Check sheet for the modelled part. Datum: model origin and axes. Units: mm. A direction names the side the tool comes from. Coordinates: 2 decimals unless noted, no trailing zeros. Write each loop counter-clockwise with the first axis right and the second up, starting at its lowest first coordinate (ties: lowest second). Pieces come first, ordered by that corner, then holes. Notation, with made-up numbers: M -8.5,-31.75 L 0.5,-31.75 A28 cw 0.5,-12.75 Z; hole C -18.5,6.25 d5. An arc over 180 degrees is marked long. Answer as CSV lines item,"result".
from build123d import *

# Parameters (mm, degrees)
BOSS_EXTRUDE1_DEPTH = 20
SKETCH2_R           = 5
CUT_EXTRUDE1_DEPTH  = 20
SKETCH3_W           = 70
SKETCH3_H           = 20
SKETCH3_R           = 5
BOSS_EXTRUDE2_DEPTH = 14.55
SKETCH4_W           = 30
SKETCH4_H           = 10
BOSS_EXTRUDE3_DEPTH = 30
SKETCH5_R           = 5
CUT_EXTRUDE2_DEPTH  = 20


with BuildPart() as part:
    # Sketch1 → Boss-Extrude1 (new body)
    with BuildSketch(Plane.XY):
        Polygon((-125, -8.78), (125, -8.78), (125, 8.78), (-125, 8.78), (-125, 5), (-100, 5), (-100, -5), (-125, -5), align=None)
    extrude(amount=BOSS_EXTRUDE1_DEPTH)

    # Sketch2 → Cut-Extrude1 (cut, symmetric)
    with BuildSketch(Plane.XZ.offset(-5)):
        with Locations((-115, 10)):
            Circle(SKETCH2_R)
        with Locations((0, 10)):
            Circle(SKETCH2_R)
        with BuildLine():
            Line((-115, 20), (-115, 22.029141536))
            Line((-115, 22.029141536), (-130, 22.029141536))
            Line((-130, 22.029141536), (-130, -2.19309391))
            Line((-130, -2.19309391), (-115, -2.19309391))
            Line((-115, -2.19309391), (-115, 0))
            ThreePointArc((-115, 0), (-125, 10), (-115, 20))
        make_face()
    extrude(amount=CUT_EXTRUDE1_DEPTH, both=True, mode=Mode.SUBTRACT)

    # Sketch3 → Boss-Extrude2 (add)
    with BuildSketch(Plane.XZ.offset(8.78)):
        with Locations((0, 10)):
            Rectangle(SKETCH3_W, SKETCH3_H)
        with Locations((0, 10)):
            Circle(SKETCH3_R, mode=Mode.SUBTRACT)
    extrude(amount=BOSS_EXTRUDE2_DEPTH)

    # Sketch4 → Boss-Extrude3 (add)
    with BuildSketch(Plane.XZ.offset(8.78)):
        with Locations((110, 10)):
            Rectangle(SKETCH4_W, SKETCH4_H)
    extrude(amount=BOSS_EXTRUDE3_DEPTH)

    # Sketch5 → Cut-Extrude2 (cut)
    with BuildSketch(Plane.XY.offset(15)):
        with Locations((110, -23.78)):
            Circle(SKETCH5_R)
    extrude(amount=-CUT_EXTRUDE2_DEPTH, mode=Mode.SUBTRACT)


solid = part.part
1) Tool access check on faces 4 (the face through (106, -20, 5)), 5 (the face through (-81, -8.78, 10)), 6 (the face through (-109.5, -5, 9.9)), 7 (the face through (-125, 7, 10)). Record the directions out of +Z, -Z, +X, -X, +Y, -Y that give a thin tool (end or side, any length) a straight path to the whole face; none if there is none.
Answer key:
face 4,"-Z, +X, -Y"
face 5,"+Z, -Z, -X, -Y"
face 6,"+Z, -Z, -X"
face 7,"-X, +Y, -Y"
2) Section check D-D, the plane y = 1. Record the boundary of the cut face in (x, z), plus the area to 3 significant figures.
Answer key:
outline,"M -100,0 L 125,0 L 125,20 L -100,20 Z; hole C 0,10 d10"
area,"4,420 mm2"
3) Mould release check, pull along Y, two halves, no side actions. Record for faces 1 (the face through (-100, 0, 10)), 2 (the face through (0, -23.33, 17)), 3 (the face through (106, -20, 15)): pulls with the +Y half, pulls with the -Y half, needs draft (parallel to the pull), parting line crosses it, or undercut.
Answer key:
face 1,"undercut"
face 2,"pulls with the -Y half"
face 3,"needs draft"
4) Section check B-B, the plane x = 0. Record the boundary of the cut face in (y, z), plus the area to 3 significant figures.
Answer key:
outline,"M -23.33,0 L 8.78,0 L 8.78,5 L -23.33,5 Z; M -23.33,15 L 8.78,15 L 8.78,20 L -23.33,20 Z"
area,"321 mm2"
5) Section check C-C, the plane z = 2.5. Record the boundary of the cut face in (x, y).
Answer key:
outline,"M -121.61,-8.78 L -35,-8.78 L -35,-23.33 L 35,-23.33 L 35,-8.78 L 125,-8.78 L 125,8.78 L -121.61,8.78 L -121.61,5 L -100,5 L -100,-5 L -121.61,-5 Z"
6) Thickness scan on line 1 along X through (y, z) = (6.5, 10.5); line 2 along Y through (x, z) = (-103, 7.25); line 3 along Y through (x, z) = (110, 11.25). Record the ranges inside material, lowest first.
Answer key:
line 1,"x = -124.99 to -119.97, -110.03 to -4.97, 4.97 to 125"
line 2,"y = -8.78 to -5, 5 to 8.78"
line 3,"y = -38.78 to -28.78, -18.78 to 8.78"
7) Section check A-A, the plane y = -11. Record the boundary of the cut face in (x, z).
Answer key:
outline,"M -35,0 L 35,0 L 35,20 L -35,20 Z; M 95,5 L 125,5 L 125,15 L 95,15 Z; hole C 0,10 d10"
8) Depth check by flat-ended pin: P1, Ø9, axis at x = 104.5, y = -19, coming from the -Z side; P2, Ø8, axis at y = -9.5, z = 5, coming from the -X side; P3, Ø2, axis at x = 56.5, y = -11.5, coming from the +Z side; P4, Ø24, axis at x = 107, y = -31, coming from the +Z side. Enter the tip coordinate at first touch or a pass-through.
Answer key:
P1,"stops at z = 5"
P2,"stops at x = -124.94"
P3,"passes through"
P4,"stops at z = 15"
